from build123d import *

# Parameters (mm, degrees)
SKETCH1_R                     = 65
SKETCH1_R_2                   = 2.5
SKETCH1_R_3                   = 50.025
SKETCH1_R_4                   = 23.5
SKETCH1_R_5                   = 37.475
SKETCH1_R_6                   = 13
LAYER_EXTRUDE_DEPTH           = 3
SKETCH1_3_R                   = 65
SKETCH1_3_R_2                 = 2.5
SKETCH1_3_R_3                 = 50.025
SKETCH1_3_R_4                 = 37.475
SKETCH1_3_R_5                 = 23.5
BEARING_SUPPORT_EXTRUDE_DEPTH = 15
SKETCH2_R                     = 5.5
CUT_EXTRUDE1_DEPTH            = 8


with BuildPart() as part:
    # Sketch1 → layer_extrude (new body)
    # profile 1 of 4: a face of its own
    with BuildSketch(Plane(origin=(0, 0, 0), x_dir=(0, 0, -1), z_dir=(1, 0, 0))):
        Circle(SKETCH1_R)
        with Locations((-49.796460718, 28.75)):
            Circle(SKETCH1_R_2, mode=Mode.SUBTRACT)
        with Locations((-49.796460718, -28.75)):
            Circle(SKETCH1_R_2, mode=Mode.SUBTRACT)
        with Locations((0, -57.5)):
            Circle(SKETCH1_R_2, mode=Mode.SUBTRACT)
        with Locations((49.796460718, -28.75)):
            Circle(SKETCH1_R_2, mode=Mode.SUBTRACT)
        with Locations((49.796460718, 28.75)):
            Circle(SKETCH1_R_2, mode=Mode.SUBTRACT)
        with Locations((0, 57.5)):
            Circle(SKETCH1_R_2, mode=Mode.SUBTRACT)
        Circle(SKETCH1_R_3, mode=Mode.SUBTRACT)
    # profile 2 of 4: a face of its own
    with BuildSketch(Plane(origin=(0, 0, 0), x_dir=(0, 0, -1), z_dir=(1, 0, 0))):
        Circle(SKETCH1_R_3)
        Circle(SKETCH1_R_4, mode=Mode.SUBTRACT)
    # profile 3 of 4: a face of its own
    with BuildSketch(Plane(origin=(0, 0, 0), x_dir=(0, 0, -1), z_dir=(1, 0, 0))):
        Circle(SKETCH1_R_5)
        Circle(SKETCH1_R_4, mode=Mode.SUBTRACT)
    # profile 4 of 4: a face of its own
    with BuildSketch(Plane(origin=(0, 0, 0), x_dir=(0, 0, -1), z_dir=(1, 0, 0))):
        Circle(SKETCH1_R_4)
        Circle(SKETCH1_R_6, mode=Mode.SUBTRACT)
    extrude(amount=LAYER_EXTRUDE_DEPTH)

    # Sketch1_3 → bearing_support_extrude (add)
    # profile 1 of 2: a face of its own
    with BuildSketch(Plane(origin=(0, 0, 0), x_dir=(0, 0, -1), z_dir=(1, 0, 0))):
        Circle(SKETCH1_3_R)
        with Locations((-49.796460718, 28.75)):
            Circle(SKETCH1_3_R_2, mode=Mode.SUBTRACT)
        with Locations((-49.796460718, -28.75)):
            Circle(SKETCH1_3_R_2, mode=Mode.SUBTRACT)
        with Locations((0, -57.5)):
            Circle(SKETCH1_3_R_2, mode=Mode.SUBTRACT)
        with Locations((49.796460718, -28.75)):
            Circle(SKETCH1_3_R_2, mode=Mode.SUBTRACT)
        with Locations((49.796460718, 28.75)):
            Circle(SKETCH1_3_R_2, mode=Mode.SUBTRACT)
        with Locations((0, 57.5)):
            Circle(SKETCH1_3_R_2, mode=Mode.SUBTRACT)
        Circle(SKETCH1_3_R_3, mode=Mode.SUBTRACT)
    # profile 2 of 2: a face of its own
    with BuildSketch(Plane(origin=(0, 0, 0), x_dir=(0, 0, -1), z_dir=(1, 0, 0))):
        Circle(SKETCH1_3_R_4)
        Circle(SKETCH1_3_R_5, mode=Mode.SUBTRACT)
    extrude(amount=BEARING_SUPPORT_EXTRUDE_DEPTH)

    # Sketch2 → Cut-Extrude1 (cut)
    with BuildSketch(Plane(origin=(15, 0, 0), x_dir=(0, 0, -1), z_dir=(1, 0, 0))):
        with Locations((0, 57.5)):
            Circle(SKETCH2_R)
        with Locations((49.796460718, 28.75)):
            Circle(SKETCH2_R)
        with Locations((49.796460718, -28.75)):
            Circle(SKETCH2_R)
        with Locations((0, -57.5)):
            Circle(SKETCH2_R)
        with Locations((-49.796460718, -28.75)):
            Circle(SKETCH2_R)
        with Locations((-49.796460718, 28.75)):
            Circle(SKETCH2_R)
    extrude(amount=-CUT_EXTRUDE1_DEPTH, mode=Mode.SUBTRACT)


solid = part.part
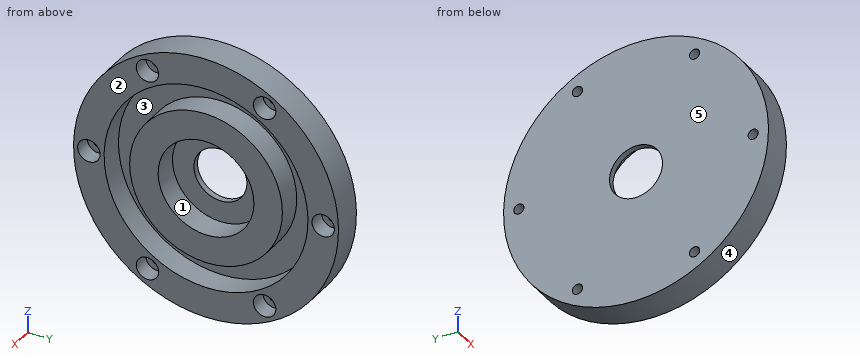
Could you check a few things on this model? Use its own coordinates, in mm. Face numbers are marked on the shaded views. A direction names the side the tool comes from. Give positions to 0.01 mm unless a question says otherwise; leave off trailing zeros. Order: outer loops, then holes, each group sorted by start corner. A loop starts at its lowest first (then second) coordinate and runs counter-clockwise, first axis right, second up.
1. For the marked faces 1 and 2, which set-ups out of +Z, -Z, +X, -X, +Y, -Y let a thin tool reach every point of the face, with its end or its side?
2. Will these pins go through, and if not, where does the flat tip stop? P1, Ø6, axis at x = 9, z = -47, coming from the +Y side; P2, Ø10, axis at y = 57.5, z = 0, coming from the +X side; P3, Ø3, axis at y = -28.75, z = -49.8, coming from the +X side; P4, Ø6, axis at x = 11, y = -5.5, coming from the -Z side.
3. Suppose I cut it at D-D (y = -28.75). List the corners of the cut face in (x, z) for me, plus the area to 3 significant figures.
4. I need wall thicknesses on L1, parallel to Y at x = 2, z = 0; L2, parallel to Y at x = 11.5, z = 0 (3 decimals); L3, parallel to Y at x = 5.5, z = 3. Which ranges of each line are inside material? Lowest first, please.
5. Suppose I cut it at A-A (x = 8.5). Give the number of separate pieces and of enclosed holes in the cut face, plus the area to 3 significant figures.
6. We'd pull the mould along Y, two halves only. Please class the marked faces 3, 4 and 5: pulls with the +Y half, pulls with the -Y half, needs draft (parallel to the pull), parting line crosses it, or undercut.
7. Suppose I cut it at B-B (y = 0). List the corners of the cut face in (x, z) for me (3 decimals).
Solved:
1. face 1: +X
1. face 2: +Z, -Z, +X, +Y, -Y
2. P1: stops at y = 47.84
2. P2: stops at x = 7
2. P3: passes through
2. P4: stops at z = -64.95
3. outline: (0, -58.3) - (15, -58.3) - (15, -55.3) - (7, -55.3) - (7, -52.3) - (0, -52.3) - close; (0, -47.3) - (7, -47.3) - (7, -44.3) - (15, -44.3) - (15, -40.94) - (3, -40.94) - (3, -24.04) - (15, -24.04) - (15, 24.04) - (3, 24.04) - (3, 40.94) - (15, 40.94) - (15, 44.3) - (7, 44.3) - (7, 47.3) - (0, 47.3) - close; (0, 52.3) - (7, 52.3) - (7, 55.3) - (15, 55.3) - (15, 58.3) - (0, 58.3) - close
3. area: 1,100 mm2
4. L1: y = -65 to -60, -55 to -13, 13 to 55, 60 to 65
4. L2: y = -65 to -63, -52 to -50.025, -37.475 to -23.5, 23.5 to 37.475, 50.025 to 52, 63 to 65
4. L3: y = -64.93 to -49.93, -37.35 to -23.31, 23.31 to 37.35, 49.93 to 64.93
5. separate pieces: 2
5. enclosed holes: 8
5. area: 7,520 mm2
6. face 3: undercut
6. face 4: parting line crosses it
6. face 5: needs draft
7. outline: (0, -65) - (15, -65) - (15, -50.025) - (3, -50.025) - (3, -37.475) - (15, -37.475) - (15, -23.5) - (3, -23.5) - (3, -13) - (0, -13) - close; (0, 13) - (3, 13) - (3, 23.5) - (15, 23.5) - (15, 37.475) - (3, 37.475) - (3, 50.025) - (15, 50.025) - (15, 65) - (0, 65) - close
